The listing builds one solid part. Answer for the finished solid, in the listing's coordinates (mm). A direction names the side the tool comes from. Give positions to 0.01 mm unless a question says otherwise; leave off trailing zeros. Loops run counter-clockwise (first coordinate to the right, second up) from the corner with the lowest first, then second, coordinate; pieces in that order, holes last. Notation, with made-up numbers: (-16, -38.5) - (28, -38.5) arc R20 ccw to (28, -4.5) - close; hole circle Ø9 at (54, -16.5). An arc over 180 degrees is marked (long way). Write item = value, one per line. Start each with the question number.
1) The part is cut by section C-C on z = 5. Write down the section's boundary in (x, y), plus the area to 3 significant figures.
2) The part is cut by section B-B on y = 10. Write down the section's boundary in (x, z), plus the area to 4 significant figures.
3) Consider probe 1 along Y at (x, z) = (-32.6, 5); probe 2 along Y at (x, z) = (-18, 4.5); probe 3 along X at (y, z) = (24.5, 13.75). Determine where each line is inside the solid, lowest interval first.
4) The part is cut by section A-A on x = -22.5. Write down the section's boundary in (y, z).
5) Flat-ended cylindrical pins translate along their axes: P1, Ø2.5, axis at y = 10.5, z = 4.5, coming from the -X side; P2, Ø0.7, axis at y = 52, z = 1.5, coming from the -X side; P3, Ø6, axis at y = 44, z = 7.5, coming from the -X side. Find the tip coordinate at first contact, or state that the pin passes through.
6) The mould has two halves that part along Z. Classify faces 1 (the flat face through (-14, 33, 0)), 2 (the flat face through (-17.6, 43.8, 12.5)), 3 (the flat face through (-14, 33, 15.5)), 4 (the flat face through (-17, 16.7, 2)): +Z half, -Z half, draft (parallel to the pull), parting line (faces both ways), or undercut.
7) Which of the six approach directions +Z, -Z, +X, -X, +Y, -Y give full straight-line access (tool end or side, diameter ignored) to faces 5 (the flat face through (-17, 18.9, 2)), 6 (the flat face through (-35, 60, 4)), 7 (the flat face through (-17, 52, 4))?
8) The part is cut by section D-D on y = 56.5. Write down the section's boundary in (x, z).
from build123d import *

# Parameters (mm, degrees)
BOSS_EXTRUDE1_DEPTH = 12.5
SKETCH2_W           = 20
SKETCH2_H           = 3.5
CUT_EXTRUDE1_DEPTH  = 10
BOSS_EXTRUDE2_DEPTH = 3
SKETCH4_R           = 2.5
CUT_EXTRUDE2_DEPTH  = 5
SKETCH5_W           = 4
SKETCH5_H           = 2.2
BOSS_EXTRUDE3_DEPTH = 4


with BuildPart() as part:
    # Sketch1 → Boss-Extrude1 (new body)
    with BuildSketch(Plane.XY):
        Polygon((0, 0), (0, 65), (-35, 65), (-35, 55), (-15, 55), (-15, 15), (-35, 15), (-35, 0), align=None)
    extrude(amount=BOSS_EXTRUDE1_DEPTH)

    # Sketch2 → Cut-Extrude1 (cut)
    with BuildSketch(Plane(origin=(0, 65, 0), x_dir=(1, 0, 0), z_dir=(0, 1, 0))):
        with Locations((-25, -10.75)):
            Rectangle(SKETCH2_W, SKETCH2_H)
    extrude(amount=-CUT_EXTRUDE1_DEPTH, mode=Mode.SUBTRACT)

    # Sketch3 → Boss-Extrude2 (add)
    with BuildSketch(Plane.XY.offset(12.5)):
        Polygon((-35, 0), (0, 0), (0, 65), (-35, 65), (-35, 52), (-18, 52), (-18, 18), (-35, 18), align=None)
    extrude(amount=BOSS_EXTRUDE2_DEPTH)

    # Sketch4 → Cut-Extrude2 (cut)
    with BuildSketch(Plane.ZY.offset(35)):
        with Locations((5, 10)):
            Circle(SKETCH4_R)
    extrude(amount=-CUT_EXTRUDE2_DEPTH, mode=Mode.SUBTRACT)

    # Sketch5 → Boss-Extrude3 (add)
    with BuildSketch(Plane.ZY.offset(15)):
        with Locations((2, 17.8)):
            Rectangle(SKETCH5_W, SKETCH5_H)
        with Locations((2, 52.2)):
            Rectangle(SKETCH5_W, SKETCH5_H)
    extrude(amount=BOSS_EXTRUDE3_DEPTH)


solid = part.part
Answer below:
q1.outline = (-35, 0) - (0, 0) - (0, 65) - (-35, 65) - (-35, 55) - (-15, 55) - (-15, 15) - (-35, 15) - (-35, 12.5) - (-30, 12.5) - (-30, 7.5) - (-35, 7.5) - close
q1.area = 1,450 mm2
q2.outline = (-35, 0) - (0, 0) - (0, 15.5) - (-35, 15.5) - (-35, 7.5) - (-30, 7.5) - (-30, 2.5) - (-35, 2.5) - close
q2.area = 517.5 mm2
q3.probe_1 = 0 to 7.5, 12.5 to 15, 55 to 65
q3.probe_2 = 0 to 15, 55 to 65
q3.probe_3 = -18 to 0
q4.outline = (0, 0) - (15, 0) - (15, 12.5) - (18, 12.5) - (18, 15.5) - (0, 15.5) - close; (52, 12.5) - (65, 12.5) - (65, 15.5) - (52, 15.5) - close; (55, 0) - (65, 0) - (65, 9) - (55, 9) - close
q5.P1 = -30
q5.P2 = -19
q5.P3 = -15
q6.face_1 = -Z half
q6.face_2 = undercut
q6.face_3 = +Z half
q6.face_4 = draft
q7.face_5 = -Z, -X
q7.face_6 = +Z, -Z, -X, +Y, -Y
q7.face_7 = -X
q8.outline = (-35, 0) - (0, 0) - (0, 15.5) - (-35, 15.5) - (-35, 12.5) - (-15, 12.5) - (-15, 9) - (-35, 9) - close
